Input: part model. Units: mm. Frame: model coordinates. Face numbers are marked on the shaded views. A direction names the side the tool comes from. Coordinates: 2 decimals unless noted, no trailing zeros. Order: outer loops, then holes, each group sorted by start corner. A loop starts at its lowest first (then second) coordinate and runs counter-clockwise, first axis right, second up. Notation, with made-up numbers: (12, 16.25) -> (32, 16.25) arc R16 ccw to (32, 23.25) -> close; hole circle Ø10 at (-15.5, -40). An arc over 180 degrees is marked (long way). Use one line per item in the form item = value. Start each with the question number.
1) Pin query (flat end, axial travel): pin 1 (8 mm diameter, centred on x = 53.5, y = 12, fed in from +Z); pin 2 (4 mm diameter, centred on y = 17.5, z = 9, fed in from +X); pin 3 (20 mm diameter, centred on x = 26.5, y = 40, fed in from +Z); pin 4 (2 mm diameter, centred on x = 16.5, y = 53.5, fed in from -Z). Return the tip coordinate at first contact, or that it passes through.
2) Ray query, line 1 along Y through (x, z) = (16.5, 4.25); line 2 along Y through (x, z) = (16.5, 3.85); line 3 along Y through (x, z) = (6.5, 5.75). Return the intervals inside material, ascending.
3) Section query C-C on z = 1.5. Count the separate pieces of the cut face and the enclosed holes in it, then the cut area to 3 significant figures.
4) Section query D-D on y = 10.5. Output: boundary loops of the cut face in (x, z).
5) Draft query along Y for the marked faces 3, 4 and 5. Return one class per face: pulls with the +Y half, pulls with the -Y half, needs draft (parallel to the pull), parting line crosses it, or undercut.
6) Section query A-A on y = 35. Output: boundary loops of the cut face in (x, z).
7) Access query for the marked faces 1 and 2. Directions: +Z, -Z, +X, -X, +Y, -Y. A direction counts if a zero-diameter tool reaches every point of the face in a straight line with its end or side. Return the directions, or none.
from build123d import *

# Parameters (mm, degrees)
SKETCH_W        = 70
SKETCH_H        = 70
PAD_DEPTH       = 4
SKETCH001_W     = 70
SKETCH001_H     = 70
PAD001_DEPTH    = 10
SKETCH002_R     = 1.7
POCKET_DEPTH    = 2
SKETCH003_R     = 1.7
POCKET001_DEPTH = 2
POCKET002_DEPTH = 3
SKETCH005_R     = 1.7
POCKET003_DEPTH = 2
POCKET004_DEPTH = 3
SKETCH007_R     = 1.7
POCKET005_DEPTH = 2
POCKET006_DEPTH = 3
SKETCH009_R     = 3
PAD002_DEPTH    = 2
SKETCH010_R     = 1.7
POCKET007_DEPTH = 2.8
SKETCH011_R     = 5
POCKET008_DEPTH = 4


with BuildPart() as part:
    # Sketch → Pad (new body)
    with BuildSketch(Plane.XY):
        with Locations((35, 35)):
            Rectangle(SKETCH_W, SKETCH_H)
    extrude(amount=PAD_DEPTH)

    # Sketch001 → Pad001 (new body)
    with BuildSketch(Plane.XY.offset(4)):
        with Locations((35, 35)):
            Rectangle(SKETCH001_W, SKETCH001_H)
        Polygon((2, 68), (2, 2), (12.5, 2), (12.5, 5), (22.5, 5), (22.5, 2), (47.5, 2), (47.5, 5), (57.5, 5), (57.5, 2), (68, 2), (68, 68), (57.5, 68), (57.5, 65), (47.5, 65), (47.5, 68), (22.5, 68), (22.5, 65), (12.5, 65), (12.5, 68), align=None, mode=Mode.SUBTRACT)
    extrude(amount=PAD001_DEPTH)

    # Sketch002 → Pocket (cut)
    with BuildSketch(Plane.YZ.offset(2)):
        with Locations((17.5, 9)):
            Circle(SKETCH002_R)
        with Locations((52.5, 9)):
            Circle(SKETCH002_R)
    extrude(amount=-POCKET_DEPTH, mode=Mode.SUBTRACT)

    # Sketch003 → Pocket001 (cut)
    with BuildSketch(Plane(origin=(68, 0, 0), x_dir=(0, -1, 0), z_dir=(-1, 0, 0))):
        with Locations((-52.5, 9)):
            Circle(SKETCH003_R)
        with Locations((-17.5, 9)):
            Circle(SKETCH003_R)
    extrude(amount=-POCKET001_DEPTH, mode=Mode.SUBTRACT)

    # Sketch004 → Pocket002 (cut)
    with BuildSketch(Plane(origin=(0, 5, 0), x_dir=(-1, 0, 0), z_dir=(0, 1, 0))):
        Polygon((-49.901924, 10.5), (-52.5, 12), (-55.098076, 10.5), (-55.098076, 7.5), (-52.5, 6), (-49.901924, 7.5), align=None)
        Polygon((-14.901924, 10.5), (-17.5, 12), (-20.098076, 10.5), (-20.098076, 7.5), (-17.5, 6), (-14.901924, 7.5), align=None)
    extrude(amount=-POCKET002_DEPTH, mode=Mode.SUBTRACT)

    # Sketch005 → Pocket003 (cut)
    with BuildSketch(Plane(origin=(0, 2, 0), x_dir=(-1, 0, 0), z_dir=(0, 1, 0))):
        with Locations((-52.5, 9)):
            Circle(SKETCH005_R)
        with Locations((-17.5, 9)):
            Circle(SKETCH005_R)
    extrude(amount=-POCKET003_DEPTH, mode=Mode.SUBTRACT)

    # Sketch006 → Pocket004 (cut)
    with BuildSketch(Plane.XZ.offset(-65)):
        Polygon((20.098076, 10.5), (17.5, 12), (14.901924, 10.5), (14.901924, 7.5), (17.5, 6), (20.098076, 7.5), align=None)
        Polygon((55.098076, 10.5), (52.5, 12), (49.901924, 10.5), (49.901924, 7.5), (52.5, 6), (55.098076, 7.5), align=None)
    extrude(amount=-POCKET004_DEPTH, mode=Mode.SUBTRACT)

    # Sketch007 → Pocket005 (cut)
    with BuildSketch(Plane.XZ.offset(-68)):
        with Locations((17.5, 9)):
            Circle(SKETCH007_R)
        with Locations((52.5, 9)):
            Circle(SKETCH007_R)
    extrude(amount=-POCKET005_DEPTH, mode=Mode.SUBTRACT)

    # Sketch008 → Pocket006 (cut)
    with BuildSketch(Plane(origin=(0, 0, 0), x_dir=(1, 0, 0), z_dir=(0, 0, -1))):
        Polygon((19.098076, -15), (16.5, -13.5), (13.901924, -15), (13.901924, -18), (16.5, -19.5), (19.098076, -18), align=None)
        Polygon((56.098076, -15), (53.5, -13.5), (50.901924, -15), (50.901924, -18), (53.5, -19.5), (56.098076, -18), align=None)
        Polygon((56.098076, -55), (56.098076, -52), (53.5, -50.5), (50.901924, -52), (50.901924, -55), (53.5, -56.5), align=None)
        Polygon((19.098076, -52), (16.5, -50.5), (13.901924, -52), (13.901924, -55), (16.5, -56.5), (19.098076, -55), align=None)
    extrude(amount=-POCKET006_DEPTH, mode=Mode.SUBTRACT)

    # Sketch009 → Pad002 (new body)
    with BuildSketch(Plane.XY.offset(4)):
        with Locations((16.5, 53.5)):
            Circle(SKETCH009_R)
        with Locations((53.5, 53.5)):
            Circle(SKETCH009_R)
        with Locations((53.5, 16.5)):
            Circle(SKETCH009_R)
        with Locations((16.5, 16.5)):
            Circle(SKETCH009_R)
    extrude(amount=PAD002_DEPTH)

    # Sketch010 → Pocket007 (cut)
    with BuildSketch(Plane.XY.offset(6)):
        with Locations((16.5, 53.5)):
            Circle(SKETCH010_R)
        with Locations((53.5, 53.5)):
            Circle(SKETCH010_R)
        with Locations((53.5, 16.5)):
            Circle(SKETCH010_R)
        with Locations((16.5, 16.5)):
            Circle(SKETCH010_R)
    extrude(amount=-POCKET007_DEPTH, mode=Mode.SUBTRACT)

    # Sketch011 → Pocket008 (cut)
    with BuildSketch(Plane.XY.offset(4)):
        with Locations((35, 35)):
            Circle(SKETCH011_R)
    extrude(amount=-POCKET008_DEPTH, mode=Mode.SUBTRACT)


solid = part.part
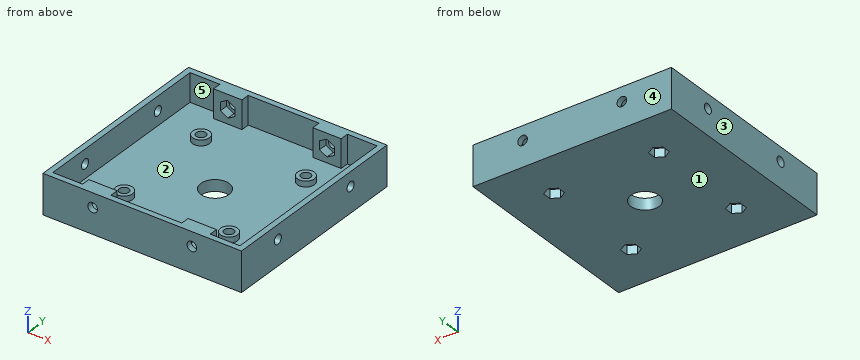
Answers below:
q1.pin_1 = 6
q1.pin_2 = 70
q1.pin_3 = 4
q1.pin_4 = 3
q2.line_1 = 0 to 5, 13.5 to 14.8, 18.2 to 19.5, 50.5 to 51.8, 55.2 to 56.5, 65 to 70
q2.line_2 = 0 to 14.8, 18.2 to 51.8, 55.2 to 70
q2.line_3 = 0 to 2, 68 to 70
q3.separate_pieces = 1
q3.enclosed_holes = 5
q3.area = 4,730 mm^2
q4.outline = (0, 0) -> (70, 0) -> (70, 14) -> (68, 14) -> (68, 4) -> (2, 4) -> (2, 14) -> (0, 14) -> close
q5.face_3 = needs draft
q5.face_4 = pulls with the +Y half
q5.face_5 = undercut
q6.outline = (0, 0) -> (30, 0) -> (30, 4) -> (2, 4) -> (2, 14) -> (0, 14) -> close; (40, 0) -> (70, 0) -> (70, 14) -> (68, 14) -> (68, 4) -> (40, 4) -> close
q7.face_1 = -Z, +X, -X, +Y, -Y
q7.face_2 = +Z
